The listing builds one solid part. Answer for the finished solid, in the listing's coordinates (mm). A direction names the side the tool comes from. Coordinates: 2 decimals unless noted, no trailing zeros. Write each loop counter-clockwise with the first axis right and the second up, starting at its lowest first coordinate (ties: lowest second). Pieces come first, ordered by that corner, then holes.
(1) For a pull along X with two mould halves and no side action, classify faces 3 (the flat face through (-9, 2, 1)), 4 (the cylindrical face through (-4.472, 3.233, 1.341)), 5 (the flat face through (0, 0, 0)), 6 (the cylindrical face through (-1.239, -0.867, 3.905)) as +X half, -X half, draft (parallel to the pull), parting line (faces both ways), or undercut.
(2) Which of the six approach directions +Z, -Z, +X, -X, +Y, -Y give full straight-line access (tool end or side, diameter ignored) to faces 1 (the cylindrical face through (-7.74, -0.867, 3.905)), 2 (the cylindrical face through (-16.395, 1.617, 0.67))?
(3) The part is cut by section C-C on x = -6. Determine the outline of the cut face in (y, z).
(4) The part is cut by section D-D on x = -18. Determine the outline of the cut face in (y, z), plus the area to 3 significant figures.
(5) Straight lines are drawn through the part: line 1 (Y direction, x = -17.5, z = 0); line 2 (X direction, y = -2.5, z = -0.5); line 3 (X direction, y = 2.25, z = -3). For each, find the intervals that lie inside material, in ascending order.
(6) Given P1, Ø3, axis at x = -9, y = 2.5, coming from the +Z side, flat-ended and moving along its own axis, determine where the tip first touches the part or whether it passes through.
from build123d import *

# Parameters (mm, degrees)
VERRUNDUNG1_R = 0.5


with BuildPart() as part:
    # Skizze1 → Rotation1 (revolve)
    with BuildSketch(Plane.XY):
        Polygon((0, 0), (-24.5, 0), (-24.5, 1.75), (-9, 1.75), (-9, 4), (-7, 4), (-7, 3.5), (-2, 3.5), (-2, 4), (0, 4), align=None)
    revolve(axis=Axis((0, 0, 0), (-1, 0, 0)))

    # Verrundung1
    verrundung1_edges = [part.edges().sort_by_distance(p)[0] for p in [
        (-24.5, -1.75, 0),
        (0, -4, 0),
        (-2, -3.5, 0),
        (-7, -3.5, 0),
        (-9, -4, 0),
    ]]
    fillet(verrundung1_edges, radius=VERRUNDUNG1_R - 0.0001)  # a hair under: the kernel refuses the full size


solid = part.part
Model answer:
1. face 3: -X half
1. face 4: undercut
1. face 5: +X half
1. face 6: draft
2. face 1: +X, -X
2. face 2: -X
3. outline: circle Ø7 at (0, 0)
4. outline: circle Ø3.5 at (0, 0)
4. area: 9.62 mm2
5. line 1: y = -1.75 to 1.75
5. line 2: x = -9 to 0
5. line 3: x = -8.93 to -6.93, -2.07 to -0.07
6. P1: stops at z = 3.85
